Could you check a few things on this model? Use its own coordinates, in mm. A direction names the side the tool comes from. Coordinates: 2 decimals unless noted, no trailing zeros. Order: outer loops, then holes, each group sorted by start corner. A loop starts at its lowest first (then second) coordinate and runs counter-clockwise, first axis right, second up.
```python
from build123d import *

# Parameters (mm, degrees)
SKETCH_3_R      = 1
EXTRUDE_1_DEPTH = 1.2


with BuildPart() as part:
    # Эскиз3 → Бобышка-Вытянуть1 (new body)
    with BuildSketch(Plane.XY):
        with BuildLine():
            Line((-3.208591813, -10.070429847), (-3.13392227, -9.838843592))
            ThreePointArc((-3.13392227, -9.838843592), (-3.772590397, -7.513749153), (-6.159272929, -7.170663716))
            ThreePointArc((-6.159272929, -7.170663716), (-7.964052136, -7.291836988), (-9.378160244, -6.16391447))
            ThreePointArc((-9.378160244, -6.16391447), (0, 10.15), (9.378160244, -6.16391447))
            ThreePointArc((9.378160244, -6.16391447), (7.964052136, -7.291836988), (6.159272929, -7.170663716))
            ThreePointArc((6.159272929, -7.170663716), (3.772590397, -7.513749153), (3.13392227, -9.838843592))
            Line((3.13392227, -9.838843592), (3.208591813, -10.070429847))
            ThreePointArc((3.208591813, -10.070429847), (4.367179244, -11.312788363), (6.063182163, -11.216074271))
            ThreePointArc((6.063182163, -11.216074271), (0, 12.75), (-6.063182163, -11.216074271))
            ThreePointArc((-6.063182163, -11.216074271), (-4.367179244, -11.312788363), (-3.208591813, -10.070429847))
        make_face()
        with Locations((-5.227775517, -9.163729839)):
            Circle(SKETCH_3_R, mode=Mode.SUBTRACT)
        with Locations((5.227775517, -9.163729839)):
            Circle(SKETCH_3_R, mode=Mode.SUBTRACT)
    extrude(amount=EXTRUDE_1_DEPTH)


solid = part.part
```
Item 1: Thinking about a two-plate mould opening in Y: for faces 1 (the face through (-4.39, -11.32, 0.59)), 2 (the face through (0.47, 12.74, 0.59)), 3 (the face through (7.989, -7.284, 0.592)), which applies, +Y half, -Y half, draft (parallel to the pull), parting line (faces both ways), or undercut?
Item 2: Suppose I cut it at B-B (y = 0). List the corners of the cut face in (x, z) for me.
Item 3: Which directions (+Z, -Z, +X, -X, +Y, -Y) give clear straight access to the entire face, cutting with the end or side of a thin tool? Please do faces 4 (the face through (-4, 10, 1.2)), 5 (the face through (-7.94, -7.3, 0.59)).
Item 4: I need wall thicknesses on line 1 (Y direction, x = 5.25, z = 0.15); line 2 (X direction, y = -9.5, z = 0.35); line 3 (Y direction, x = 4.75, z = 1.05). Which ranges of each line are inside material? Lowest first, please.
Item 5: Suppose I cut it at A-A (x = 7.75). List the corners of the cut face in (y, z) for me.
Item 6: Suppose I cut it at C-C (x = -5). List the corners of the cut face in (y, z) for me.
Item 7: Suppose I cut it at D-D (z = 0.6). List the corners of the cut face in (x, y) for me, and give its area (3 significant figures).
Geometry results:
1. face 1: -Y half
1. face 2: parting line
1. face 3: undercut
2. outline: (-12.75, 0) - (-10.83, 0) - (-10.83, 1.2) - (-12.75, 1.2) - close; (10.83, 0) - (12.75, 0) - (12.75, 1.2) - (10.83, 1.2) - close
3. face 4: +Z, +X, -X, +Y, -Y
3. face 5: +Z, -Z
4. line 1: y = -11.45 to -10.16, -8.16 to -6.96, 8.8 to 11.62
4. line 2: x = -8.5 to -6.17, -4.29 to -3.05, 3.05 to 4.29, 6.17 to 8.5
4. line 3: y = -11.42 to -10.04, -8.29 to -7.02, 9.06 to 11.83
5. outline: (-10.12, 0) - (-7.35, 0) - (-7.35, 1.2) - (-10.12, 1.2) - close; (6.89, 0) - (10.12, 0) - (10.12, 1.2) - (6.89, 1.2) - close
6. outline: (-11.45, 0) - (-10.14, 0) - (-10.14, 1.2) - (-11.45, 1.2) - close; (-8.19, 0) - (-6.98, 0) - (-6.98, 1.2) - (-8.19, 1.2) - close; (8.93, 0) - (11.73, 0) - (11.73, 1.2) - (8.93, 1.2) - close
7. outline: (-9.38, -6.16) arc R10.85 cw (long way) to (9.38, -6.16) arc R2.5 cw to (6.16, -7.17) arc R2.2 ccw to (3.13, -9.84) - (3.21, -10.07) arc R2 ccw to (6.06, -11.22) arc R12.75 ccw (long way) to (-6.06, -11.22) arc R2 ccw to (-3.21, -10.07) - (-3.13, -9.84) arc R2.2 ccw to (-6.16, -7.17) arc R2.5 cw to start; hole circle Ø2 at (-5.23, -9.16); hole circle Ø2 at (5.23, -9.16)
7. area: 149 mm2
